Design review of the part built by this model. Coordinates are the model's own, in mm. Face numbers are marked on the shaded views. Coordinates: 2 decimals unless noted, no trailing zeros. Write each loop counter-clockwise with the first axis right and the second up, starting at its lowest first coordinate (ties: lowest second). Pieces come first, ordered by that corner, then holes. Notation, with made-up numbers: (-6.75, 1.5) - (-1.75, 1.5) arc R34 cw to (-1.75, 40.5) - close; hole circle Ø10 at (7.5, -0.5). An arc over 180 degrees is marked (long way). Answer as CSV lines item,"result". Start each with the question number.
Q1. We need section B-B (y = 9.25). Write out the cut boundary in (x, z), plus the area to 3 significant figures.
Q2. For line 1 along Z through (x, y) = (19.5, 1.5); line 2 along X through (y, z) = (4, -11), list the stretches that pass through material, from the lowest coordinate up. Write a range as [from, to].
Q3. We need section C-C (z = -13.5). Write out the cut boundary in (x, y), plus the area to 3 significant figures.
Q4. Mouldability with a two-part tool opening along X and no side actions: class the marked faces 1, 2 and 3 as pulls with the +X half, pulls with the -X half, needs draft (parallel to the pull), parting line crosses it, or undercut.
Q5. We need section A-A (x = -19.5). Write out the cut boundary in (y, z).
Q6. Clearance check with flat-ended pins moving along their axes: pin 1 (1.5 mm diameter, centred on x = -10, y = 19.5, fed in from -Z); pin 2 (3.5 mm diameter, centred on x = 8.5, z = -19.5, fed in from +Y); pin 3 (8 mm diameter, centred on x = -11.5, y = 9, fed in from +Z); pin 4 (22.5 mm diameter, centred on x = -4.5, z = 6, fed in from +Y). State where each tip first meets the part, or that it passes through.
Q7. We need section D-D (x = -9). Write out the cut boundary in (y, z).
from build123d import *

# Parameters (mm, degrees)
SKETCH1_W           = 45
SKETCH1_H           = 45
SKETCH1_R           = 1.5
BOSS_EXTRUDE1_DEPTH = 2
BOSS_EXTRUDE2_DEPTH = 25


with BuildPart() as part:
    # Sketch1 → Boss-Extrude1 (new body)
    with BuildSketch(Plane(origin=(0, 0, 0), x_dir=(1, 0, 0), z_dir=(0, 1, 0))):
        Rectangle(SKETCH1_W, SKETCH1_H)
        with Locations((-19.5, 19.5)):
            Circle(SKETCH1_R, mode=Mode.SUBTRACT)
        with Locations((19.5, 19.5)):
            Circle(SKETCH1_R, mode=Mode.SUBTRACT)
        with Locations((-19.5, -19.5)):
            Circle(SKETCH1_R, mode=Mode.SUBTRACT)
        with Locations((19.5, -19.5)):
            Circle(SKETCH1_R, mode=Mode.SUBTRACT)
    extrude(amount=BOSS_EXTRUDE1_DEPTH)

    # Sketch2 → Boss-Extrude2 (add)
    with BuildSketch(Plane(origin=(0, 2, 0), x_dir=(1, 0, 0), z_dir=(0, 1, 0))):
        Polygon((10, 7.5), (12.5, 7.5), (12.5, 22.5), (10, 22.5), (10, 16.2), (7, 16.2), (7, 22.5), (5.5, 22.5), (5.5, 16.2), (2.5, 16.2), (2.5, 22.5), (1, 22.5), (1, 16.2), (-2, 16.2), (-2, 22.5), (-3.5, 22.5), (-3.5, 16.2), (-6.5, 16.2), (-6.5, 22.5), (-8, 22.5), (-8, 16.2), (-11, 16.2), (-11, 22.5), (-12.5, 22.5), (-12.5, 7.5), (-11, 7.5), (-11, 15), (10, 15), align=None)
    extrude(amount=BOSS_EXTRUDE2_DEPTH)


solid = part.part
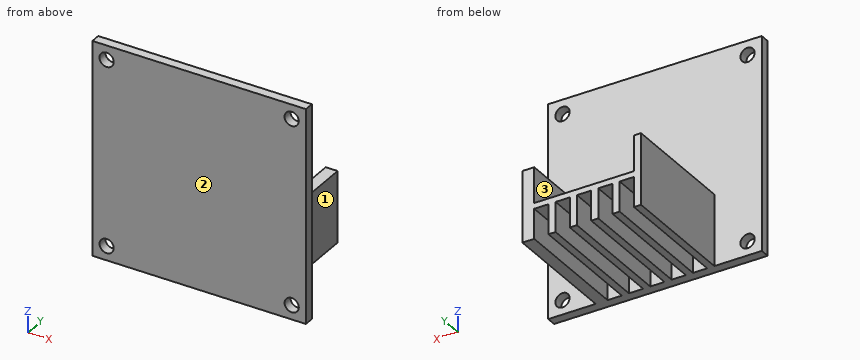
Results list:
1,outline,"(-12.5, -22.5) - (-11, -22.5) - (-11, -16.2) - (-8, -16.2) - (-8, -22.5) - (-6.5, -22.5) - (-6.5, -16.2) - (-3.5, -16.2) - (-3.5, -22.5) - (-2, -22.5) - (-2, -16.2) - (1, -16.2) - (1, -22.5) - (2.5, -22.5) - (2.5, -16.2) - (5.5, -16.2) - (5.5, -22.5) - (7, -22.5) - (7, -16.2) - (10, -16.2) - (10, -22.5) - (12.5, -22.5) - (12.5, -7.5) - (10, -7.5) - (10, -15) - (-11, -15) - (-11, -7.5) - (-12.5, -7.5) - close"
1,area,"123 mm2"
2,line 1,"z = [-22.5, -21], [-18, 18], [21, 22.5]"
2,line 2,"x = [-12.5, -11], [10, 12.5]"
3,outline,"(-22.5, 0) - (22.5, 0) - (22.5, 2) - (12.5, 2) - (12.5, 27) - (10, 27) - (10, 2) - (-11, 2) - (-11, 27) - (-12.5, 27) - (-12.5, 2) - (-22.5, 2) - close"
3,area,"190 mm2"
4,face 1,"pulls with the +X half"
4,face 2,"needs draft"
4,face 3,"undercut"
5,outline,"(0, -22.5) - (2, -22.5) - (2, -21) - (0, -21) - close; (0, -18) - (2, -18) - (2, 18) - (0, 18) - close; (0, 21) - (2, 21) - (2, 22.5) - (0, 22.5) - close"
6,pin 1,"stops at z = -16.2"
6,pin 2,"stops at y = 27"
6,pin 3,"stops at z = -7.5"
6,pin 4,"stops at y = 2"
7,outline,"(0, -22.5) - (2, -22.5) - (2, -16.2) - (27, -16.2) - (27, -15) - (2, -15) - (2, 22.5) - (0, 22.5) - close"
